Work out the finished part from the listing and answer in its coordinate system (mm). A direction names the side the tool comes from. Round coordinates to 2 decimals unless told otherwise and drop trailing zeros. Order: outer loops, then holes, each group sorted by start corner. A loop starts at its lowest first (then second) coordinate and runs counter-clockwise, first axis right, second up.
Autodesk Inventor part; units mm, degrees
ref_plane "YZ Plane" through (0, 0, 0) normal (1, 0, 0) x (0, 1, 0)
ref_plane "XZ Plane" through (0, 0, 0) normal (0, 1, 0) x (-1, 0, 0)
ref_plane "XY Plane" through (0, 0, 0) normal (0, 0, 1) x (1, 0, 0)
sketch "Sketch1" plane through (0, 0, 0) normal (0, 1, 0) x (-1, 0, 0)
  line L0 (10, 5) -> (-10, 5)
  line L1 (-10, 5) -> (-10, -5)
  line L2 (-10, -5) -> (10, -5)
  line L3 (10, -5) -> (10, 5)
  line L4 (10, 5) -> (-10, -5) construction
  line L5 (-10, 5) -> (10, -5) construction
  point P0 (0, 0)
  dimension "d0" = 20
  dimension "d1" = 10
extrude "Extrusion1" add sketch "Sketch1" along normal blind 2
sketch "Sketch2" plane through (0, 2, 0) normal (0, 1, 0) x (1, 0, 0)
  line L0 (-10, -5) -> (10, -5) construction
  line L1 (10, -5) -> (10, 5) construction
  line L2 (10, 5) -> (-10, 5) construction
  line L3 (-10, 5) -> (-10, -5) construction
  line L4 (-10, 5) -> (-10, -5) construction
  line L5 (-10, 0) -> (10, 0) construction
  point P0 (0, 0)
ref_plane "Work Plane1" through (-10, 2, 0) normal (0, 0, 1) x (1, 0, 0)
sketch "Sketch3" plane through (-10, 2, 0) normal (0, 0, 1) x (1, 0, 0)
  line L0 (0, 0) -> (20, 0) construction
  line L1 (2.5, 0) -> (4, 0)
  line L2 (0, 0) -> (20, 0)
  line L3 (16, 0) -> (17.5, 0)
  arc A0 (16, 0) -> (12.0028, 5.6558) centre (10, 0) ccw
  arc A1 (7.9972, 5.6558) -> (4, 0) centre (10, 0) ccw
  arc A2 (17.5, 0) -> (12.5036, 7.0698) centre (10, 0) ccw
  arc A3 (7.4964, 7.0698) -> (2.5, 0) centre (10, 0) ccw
  line L4 (10, 0) -> (10, 7.5) construction
  line L5 (10, 0) -> (12.5036, 7.0698)
  line L6 (10, 0) -> (10, 7.5) construction
  line L7 (10, 0) -> (10, 7.5) construction
  line L8 (10, 0) -> (7.4964, 7.0698)
  line L9 (10, 0) -> (10, 7.5) construction
  point P0 (10, -2)
  point P1 (7.1395, 6.9331)
  point P2 (12.8605, 6.9331)
  point P3 (7.7742, 5.5719)
  point P4 (12.2258, 5.5719)
  point P5 (6.1541, 6.4389)
  point P6 (13.8459, 6.4389)
  dimension "d14" = 19.5
  dimension "d16" = 19.5
extrude "Extrusion2" add sketch "Sketch3" along normal blind 2 and the other way blind 2 contours A3 L8 A1 L1 | A0 L5 A2 L2
fillet "Fillet1" radius 2 2 edges at (-2.5036, 9.0698, 0) (2.5036, 9.0698, 0)
fillet "Fillet2" radius 1 8 edges at (0, 2, 5) (10, 2, 0) (0, 2, -5) (-10, 2, 0) (10, 1, -5) (-10, 1, -5) (-10, 1, 5) (10, 1, 5)
fillet "Fillet4" radius 2 2 edges at (-6, 2, 0) (6, 2, 0)
fillet "Fillet4" radius 1 6 edges at (6.75, 2, 2) (7.5, 2, 0) (6.75, 2, -2) (-6.75, 2, 2) (-7.5, 2, 0) (-6.75, 2, -2)
properties part number "cable_holder"
Item 1: For a pull along X with two mould halves and no side action, classify faces 5 (the face through (0.126, 1.715, 4.699)), 6 (the face through (-7.78, 2.25, 0.04)), 7 (the face through (5.18, 2.97, 0.04)), 8 (the face through (-3.301, 8.274, 0.028)) as released by +X, released by -X, zero draft, split by the parting line, or undercut.
Item 2: Find section C-C (z = 1). Write down the section's boundary in (x, y), plus the area to 3 significant figures.
Item 3: A tool of negligible diameter and unlimited length cuts with its end or side. For faces 1 (the face through (0, 2, 0)), 2 (the face through (-9.715, 0.507, 4.699)), 3 (the face through (-5, 6, -2)), 4 (the face through (-5, 6, 2)), from which of +Z, -Z, +X, -X, +Y, -Y can it reach the whole face along a straight path? Write none if from no direction.
Item 4: Find the intervals of material crossed by line 1 along X through (y, z) = (3, 0.75); line 2 along Z through (x, y) = (5.5, 5.75); line 3 along Y through (x, z) = (0.25, 3.5), in increasing order.
Item 5: Find section B-B (x = 5). Write down the section's boundary in (y, z), plus the area to 3 significant figures.
Item 6: Given pin 1 (4 mm diameter, centred on y = 6, z = 3, fed in from +X); pin 2 (1.6 mm diameter, centred on x = -5, y = 6, fed in from +Z); pin 3 (2 mm diameter, centred on y = 4, z = -2, fed in from +X), each flat-ended and moving along its own axis, determine where each tip first touches the part or whether it passes through.
Item 7: Find section D-D (x = 7). Write down the section's boundary in (y, z).
Item 8: Find section A-A (y = 3.75). Write down the section's boundary in (x, z), plus the area to 3 significant figures.
Model answer:
1. face 5: zero draft
1. face 6: released by -X
1. face 7: undercut
1. face 8: undercut
2. outline: (-10, 0) - (10, 0) - (10, 1) arc R1 ccw to (9, 2) - (8.44, 2) arc R1 cw to (7.45, 2.88) arc R7.5 ccw to (4.71, 7.84) arc R2 ccw to (2, 7.66) arc R6 cw to (5.2, 5) arc R2 cw to (3.46, 2) - (-3.46, 2) arc R2 cw to (-5.2, 5) arc R6 cw to (-2, 7.66) arc R2 ccw to (-4.71, 7.84) arc R7.5 ccw to (-7.45, 2.88) arc R1 cw to (-8.44, 2) - (-9, 2) arc R1 ccw to (-10, 1) - close
2. area: 66.3 mm2
3. face 1: none
3. face 2: +Z, -X, +Y, -Y
3. face 3: -Z, +X, -X, +Y
3. face 4: +Z, +X, -X, +Y
4. line 1: x = -7.43 to -5.2, 5.2 to 7.43
4. line 2: z = -2 to 2
4. line 3: y = 0 to 2
5. outline: (0, -5) - (1, -5) arc R1 ccw to (2, -4) - (2, -3) arc R1 cw to (2.72, -2.04) - (2.72, 2.04) arc R1 cw to (2, 3) - (2, 4) arc R1 ccw to (1, 5) - (0, 5) - close; (5.32, -2) - (7.59, -2) - (7.59, 2) - (5.32, 2) - close
5. area: 32.0 mm2
6. pin 1: stops at x = 7.15
6. pin 2: stops at z = 2
6. pin 3: stops at x = 7.43
7. outline: (0, -5) - (1, -5) arc R1 ccw to (2, -4) - (2, -3) arc R1 cw to (3, -2) - (4.69, -2) - (4.69, 2) - (3, 2) arc R1 cw to (2, 3) - (2, 4) arc R1 ccw to (1, 5) - (0, 5) - close
8. outline: (-7.29, -2) - (-5.45, -2) - (-5.45, 2) - (-7.29, 2) - close; (5.45, -2) - (7.29, -2) - (7.29, 2) - (5.45, 2) - close
8. area: 14.8 mm2
